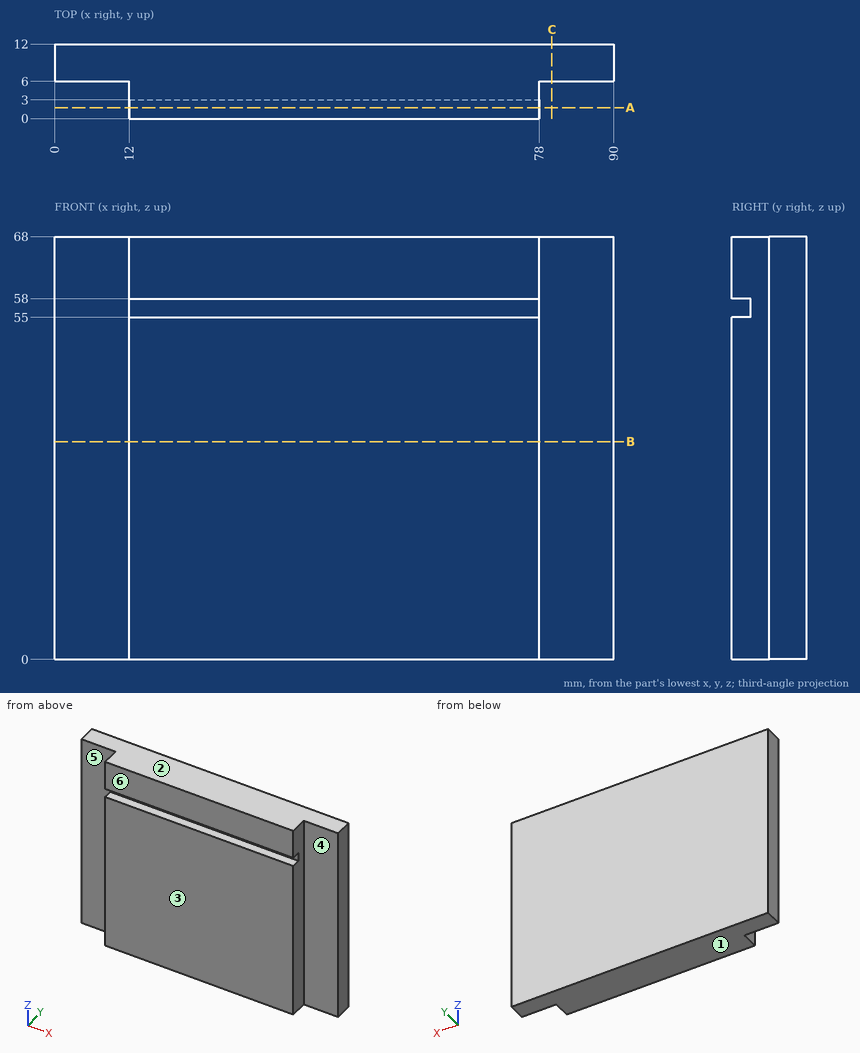
Verification items for this drawing (mm, ordinates from the low corner). A direction names the side the tool comes from. Give positions to 0.01 mm unless a question says otherwise; leave off trailing zeros. Loops run counter-clockwise (first coordinate to the right, second up) from the corner with the lowest first, then second, coordinate; pieces in that order, holes last.
(1) Section check A-A on y = 1.75. Record the cut outline in (x, z).
From the geometry:
outline: (12, 0) - (78, 0) - (78, 55) - (12, 55) - close; (12, 58) - (78, 58) - (78, 68) - (12, 68) - close
(2) Thickness scan on L1, parallel to Z at x = 15, y = 1.25; L2, parallel to X at y = 1.25, z = 48.5; L3, parallel to Y at x = 8.5, z = 64. Record the ranges inside material, lowest first.
From the geometry:
L1: z = 0 to 55, 58 to 68
L2: x = 12 to 78
L3: y = 6 to 12
(3) Release check for a two-part mould opening along Z. For the marked faces 1, 2 and 3 record: released by +Z, released by -Z, zero draft, split by the parting line, or undercut.
From the geometry:
face 1: released by -Z
face 2: released by +Z
face 3: zero draft
(4) Section check C-C on x = 80. Record the cut outline in (y, z).
From the geometry:
outline: (6, 0) - (12, 0) - (12, 68) - (6, 68) - close
(5) Section check B-B on z = 35. Record the cut outline in (x, y).
From the geometry:
outline: (0, 6) - (12, 6) - (12, 0) - (78, 0) - (78, 6) - (90, 6) - (90, 12) - (0, 12) - close
(6) Depth check by flat-ended pin: pin 1 Ø6 at (x, z) = (6, 22) entering from -Y; pin 2 Ø3 at (y, z) = (1.5, 28) entering from +X; pin 3 Ø6.5 at (y, z) = (2.5, 41.5) entering from -X. Enter the tip coordinate at first touch or a pass-through.
From the geometry:
pin 1: stops at y = 6
pin 2: stops at x = 78
pin 3: stops at x = 12
(7) Set-up check for the marked faces 4, 5 and 6: record each of +Z, -Z, +X, -X, +Y, -Y from which the full face is reachable in a straight line by a thin tool's end or side.
From the geometry:
face 4: +Z, -Z, +X, -Y
face 5: +Z, -Z, -X, -Y
face 6: +Z, -Z, +X, -X, -Y
